```python
from build123d import *

# Parameters (mm, degrees)
F5_DEPTH = 175


with BuildPart() as f3:
    # F3: sweep along a path in F0
    with BuildLine(Plane.YZ) as f3_path:
        Line((0, 0), (-46.1925436563, 527.9831899886))
        Line((-46.1925436563, 527.9831899886), (-310.0377043777, 904.7931303616))
        Line((-310.0377043777, 904.7931303616), (-227.2156099449, 1213.8893947741))
    # F2 (on line) → F3 (sweep)
    with BuildSketch(Plane(origin=(0, 0, 0), x_dir=(1, 0, 0), z_dir=(0, 0.0871557427, -0.9961946981))):
        with BuildLine():
            ThreePointArc((-12.5, -7.5), (-11.0355339059, -11.0355339059), (-7.5, -12.5))
            Line((-7.5, -12.5), (7.5, -12.5))
            ThreePointArc((7.5, -12.5), (11.0355339059, -11.0355339059), (12.5, -7.5))
            Line((12.5, -7.5), (12.5, 7.5))
            ThreePointArc((12.5, 7.5), (11.0355339059, 11.0355339059), (7.5, 12.5))
            Line((7.5, 12.5), (-7.5, 12.5))
            ThreePointArc((-7.5, 12.5), (-11.0355339059, 11.0355339059), (-12.5, 7.5))
            Line((-12.5, 7.5), (-12.5, -7.5))
        make_face()
        with BuildLine():
            ThreePointArc((10, -7.5), (9.267766953, -9.267766953), (7.5, -10))
            Line((7.5, -10), (-7.5, -10))
            ThreePointArc((-7.5, -10), (-9.267766953, -9.267766953), (-10, -7.5))
            Line((-10, -7.5), (-10, 7.5))
            ThreePointArc((-10, 7.5), (-9.267766953, 9.267766953), (-7.5, 10))
            Line((-7.5, 10), (7.5, 10))
            ThreePointArc((7.5, 10), (9.267766953, 9.267766953), (10, 7.5))
            Line((10, 7.5), (10, -7.5))
        make_face(mode=Mode.SUBTRACT)
    sweep(path=f3_path.line, transition=Transition.RIGHT)

    # F4 (on face) → F5 (join)
    with BuildSketch(Plane(origin=(-12.5, 0, 0), x_dir=(0, -1, 0), z_dir=(-1, 0, 0))):
        with BuildLine():
            Line((234.4600536421, 1215.8305376123), (219.9711662478, 1211.9482519358))
            ThreePointArc((219.9711662478, 1211.9482519358), (216.9351344544, 1209.6186228043), (216.4356323418, 1205.8245275788))
            Line((216.4356323418, 1205.8245275788), (220.3179180184, 1191.3356401845))
            ThreePointArc((220.3179180184, 1191.3356401845), (222.6475471498, 1188.2996083911), (226.4416423753, 1187.8001062786))
            Line((226.4416423753, 1187.8001062786), (240.9305297697, 1191.6823919551))
            ThreePointArc((240.9305297697, 1191.6823919551), (243.9665615631, 1194.0120210866), (244.4660636756, 1197.8061163121))
            Line((244.4660636756, 1197.8061163121), (240.5837779991, 1212.2950037064))
            ThreePointArc((240.5837779991, 1212.2950037064), (238.2541488676, 1215.3310354998), (234.4600536421, 1215.8305376123))
        make_face()
        with BuildLine():
            ThreePointArc((235.1071012549, 1213.4157230466), (237.0041488676, 1213.1659719903), (238.1689634333, 1211.6479560936))
            Line((238.1689634333, 1211.6479560936), (242.0512491099, 1197.1590686993))
            ThreePointArc((242.0512491099, 1197.1590686993), (241.8014980536, 1195.2620210866), (240.2834821569, 1194.0972065208))
            Line((240.2834821569, 1194.0972065208), (225.7945947626, 1190.2149208443))
            ThreePointArc((225.7945947626, 1190.2149208443), (223.8975471498, 1190.4646719006), (222.7327325841, 1191.9826877973))
            Line((222.7327325841, 1191.9826877973), (218.8504469076, 1206.4715751916))
            ThreePointArc((218.8504469076, 1206.4715751916), (219.1001979638, 1208.3686228043), (220.6182138605, 1209.5334373701))
            Line((220.6182138605, 1209.5334373701), (235.1071012549, 1213.4157230466))
        make_face(mode=Mode.SUBTRACT)
    extrude(amount=F5_DEPTH)

    # F6: F3 across face


with BuildPart() as f3_1:
    add(f3.part)
    add(f3.part.mirror(Plane(origin=(-187.5, -230.4508480087, 1201.8153219455), x_dir=(0, -1, 0), z_dir=(-1, 0, 0))))


solid = f3_1.part
```
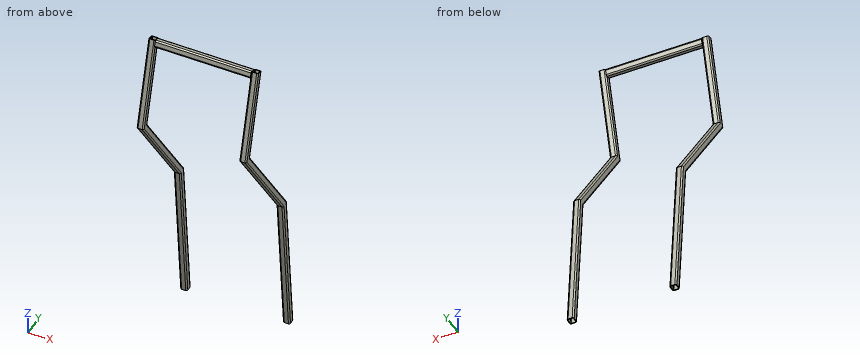
The model under review builds one solid part; all positions refer to its coordinate system, in mm. Round coordinates to 2 decimals unless told otherwise and drop trailing zeros. Loops run counter-clockwise (first coordinate to the right, second up) from the corner with the lowest first, then second, coordinate; pieces in that order, holes last. Notation, with made-up numbers: (4, 55) -> (40, 55) arc R27 ccw to (40, 78) -> close; hole circle Ø7 at (-38, 87.5). An arc over 180 degrees is marked (long way). Answer in a Markdown table with one row per item.
1) Wall thickness on line 1 along X through (y, z) = (-11, 85): over which ranges is the line inside the solid? List them lowest first.
Taken from the geometry:
| item | result |
|---|---|
| line 1 | x = -387.5 to -385, -365 to -362.5, -12.5 to -10, 10 to 12.5 |
2) Consider section B-B, the plane y = -169. Count the separate pieces of the cut face and the enclosed holes in it, plus the area to 3 significant figures.
Taken from the geometry:
| item | result |
|---|---|
| separate pieces | 2 |
| enclosed holes | 2 |
| area | 728 mm² |
3) For pin 1 Ø8 at (y, z) = (-221, 1203.5) entering from +X; pin 2 Ø3 at (y, z) = (-240.5, 1202) entering from -X; pin 3 Ø4 at (x, y) = (-231, -221) entering from -Z, all flat-tipped, find the tip position at first contact; note any pin that passes through.
Taken from the geometry:
| item | result |
|---|---|
| pin 1 | stops at x = 12.5 |
| pin 2 | stops at x = -387.44 |
| pin 3 | stops at z = 1188.11 |
4) Consider section A-A, the plane x = -259.5. Write out the cut boundary in (y, z) (3 decimals), plus the area to 3 significant figures.
Taken from the geometry:
| item | result |
|---|---|
| outline | (-244.466, 1197.806) arc R5 ccw to (-240.931, 1191.682) -> (-226.442, 1187.8) arc R5 ccw to (-220.318, 1191.336) -> (-216.436, 1205.825) arc R5 ccw to (-219.971, 1211.948) -> (-234.46, 1215.831) arc R5 ccw to (-240.584, 1212.295) -> close; hole (-242.051, 1197.159) arc R2.5 ccw to (-240.283, 1194.097) -> (-225.795, 1190.215) arc R2.5 ccw to (-222.733, 1191.983) -> (-218.85, 1206.472) arc R2.5 ccw to (-220.618, 1209.533) -> (-235.107, 1213.416) arc R2.5 ccw to (-238.169, 1211.648) -> close |
| area | 209 mm² |
